Design review of the part built by this model. Coordinates are the model's own, in mm. A direction names the side the tool comes from. Give positions to 0.01 mm unless a question says otherwise; leave off trailing zeros. Write each loop counter-clockwise with the first axis right and the second up, starting at its lowest first coordinate (ties: lowest second). Pieces come first, ordered by that corner, then holes. Notation, with made-up numbers: M -27,56 L -12,56 A19 ccw -12,90 Z; hole C 42.5,7 d11. An arc over 180 degrees is marked long. Use a Markdown table: item, result. Add a question column.
Autodesk Inventor part; units mm, degrees
ref_plane "Start plane" through (0, 0, 0) normal (0, 0, 1) x (1, 0, 0)
ref_plane "End plane" through (0, 0, 685) normal (0, 0, 1) x (1, 0, 0)
ref_plane "Work Plane4" through (0, 0, 342.5) normal (-1, 0, 0) x (0, 0, 1)
ref_plane "Start plane" through (0, 0, 0) normal (0, 0, 1) x (1, 0, 0)
ref_plane "End plane" through (0, 0, 685) normal (0, 0, 1) x (1, 0, 0)
sketch "Sketch" plane through (0, 0, 0) normal (0, 0, 1) x (1, 0, 0)
  line L0 (-17.5, -13.5) -> (-17.5, 13.5)
  line L1 (-13.5, 17.5) -> (13.5, 17.5)
  line L2 (17.5, 13.5) -> (17.5, -13.5)
  line L3 (13.5, -17.5) -> (-13.5, -17.5)
  arc A0 (-17.5, -13.5) -> (-13.5, -17.5) centre (-13.5, -13.5) ccw
  arc A1 (-13.5, 17.5) -> (-17.5, 13.5) centre (-13.5, 13.5) ccw
  arc A2 (17.5, 13.5) -> (13.5, 17.5) centre (13.5, 13.5) ccw
  arc A3 (13.5, -17.5) -> (17.5, -13.5) centre (13.5, -13.5) ccw
  arc A4 (-13.5, 15.5) -> (-15.5, 13.5) centre (-13.5, 13.5) ccw
  line L4 (-13.5, 15.5) -> (13.5, 15.5)
  arc A5 (15.5, 13.5) -> (13.5, 15.5) centre (13.5, 13.5) ccw
  line L5 (15.5, 13.5) -> (15.5, -13.5)
  arc A6 (13.5, -15.5) -> (15.5, -13.5) centre (13.5, -13.5) ccw
  line L6 (13.5, -15.5) -> (-13.5, -15.5)
  arc A7 (-15.5, -13.5) -> (-13.5, -15.5) centre (-13.5, -13.5) ccw
  line L7 (-15.5, -13.5) -> (-15.5, 13.5)
  line L8 (0, 25.6598) -> (0, -25.6598) construction
  line L9 (-25.6598, 0) -> (25.6598, 0) construction
  dimension "d7" = 4
  dimension "d10" = 35
  dimension "d11" = 35
  dimension "d12" = 2
  dimension "d15" = 17.5
  dimension "d16" = 17.5
extrude "Body" add sketch "Sketch" along normal up to surface (685 mm away) from surface at 0
sketch "Sketch3" plane through (0, 0, 0) normal (0, 0, 1) x (1, 0, 0)
  line L0 (0, 0) -> (10, 0)
ref_plane "Work Plane3" through (0, 0, 0) normal (0, -1, 0) x (1, 0, 0)
sketch "Sketch4" plane through (0, 0, 0) normal (0, -1, 0) x (1, 0, 0)
  line L0 (-2, 0) -> (12, 0)
  line L1 (-2, 685) -> (12, 685)
  dimension "d18" = 685
ref_plane "Work Plane4" through (0, 0, 342.5) normal (-1, 0, 0) x (0, 0, 1)
ref_plane "Work Plane5" through (-395, 0, 342.5) normal (-1, 0, 0) x (0, 0, 1)
ref_plane "Work Plane6" through (-197.5, 0, 342.5) normal (-1, 0, 0) x (0, 0, 1)
sketch "Sketch5" plane through (-197.5, 0, 342.5) normal (-1, 0, 0) x (0, 0, 1)
  arc A0 (-17.5, -13.5) -> (-13.5, -17.5) centre (-13.5, -13.5) ccw
  line L0 (-17.5, -13.5) -> (-17.5, 13.5)
  arc A1 (-13.5, 17.5) -> (-17.5, 13.5) centre (-13.5, 13.5) ccw
  line L1 (-13.5, 17.5) -> (13.5, 17.5)
  arc A2 (17.5, 13.5) -> (13.5, 17.5) centre (13.5, 13.5) ccw
  line L2 (17.5, 13.5) -> (17.5, -13.5)
  arc A3 (13.5, -17.5) -> (17.5, -13.5) centre (13.5, -13.5) ccw
  line L3 (13.5, -17.5) -> (-13.5, -17.5)
  arc A4 (-13.5, 15.5) -> (-15.5, 13.5) centre (-13.5, 13.5) ccw
  line L4 (-13.5, 15.5) -> (13.5, 15.5)
  arc A5 (15.5, 13.5) -> (13.5, 15.5) centre (13.5, 13.5) ccw
  line L5 (15.5, 13.5) -> (15.5, -13.5)
  arc A6 (13.5, -15.5) -> (15.5, -13.5) centre (13.5, -13.5) ccw
  line L6 (13.5, -15.5) -> (-13.5, -15.5)
  arc A7 (-15.5, -13.5) -> (-13.5, -15.5) centre (-13.5, -13.5) ccw
  line L7 (-15.5, -13.5) -> (-15.5, 13.5)
extrude "Extrusion2" cut sketch "Sketch5" along normal up to surface (395 mm away) from surface at -197.5 contours L0 A1 L1 A2 L2 A3 L3 A0 | L4 A5 L5 A6 L6 A7 L7 A4
equation "\"d7\" = G_IR"
equation "\"d10\" = G_H"
equation "\"d11\" = G_W"
equation "\"d12\" = G_T"
equation "\"d15\" = 0.5 * d10"
equation "\"d16\" = 0.5 * d11"
equation "\"d3\" = G_L"
equation "\"G_W\" = 35"
equation "\"G_H\" = 35"
equation "\"G_T\" = 2"
equation "\"G_IR\" = 4"
equation "\"G_L\" = d18"
equation "\"G_OFFSET_START\" = 0"
equation "\"G_OFFSET_END\" = 0"
equation "\"d14\" = G_OFFSET_END + B_L"
equation "\"B_L\" = 685"
properties part number "AS 1163 - C350L0 35x35x2.0 SHS - 685" material "Steel, Mild"
(1) Add section C-C on z = 191. Give the boundary of the cut face in (x, y), then the cut area to 3 significant figures.
(2) For pin 1 (1.6 mm diameter, centred on y = -17, z = 336.5, fed in from -X); pin 2 (1 mm diameter, centred on x = -16, y = 5, fed in from -Z); pin 3 (5 mm diameter, centred on y = 5, z = 350, fed in from -X), all flat-tipped, find the tip position at first contact; note any pin that passes through.
(3) Add section B-B on x = 8. Give the boundary of the cut face in (y, z), then the cut area to 3 significant figures.
(4) Add section A-A on y = -0.5. Give the boundary of the cut face in (x, z).
(5) The part is to be moulded in two halves that separate along Y. For faces 3 (the flat face through (-16, 3, 0)), 4 (the flat face through (3, 17.5, 338)), 5 (the flat face through (0.2, -15.5, 337.7)), say which applies: released by +Y, released by -Y, zero draft, split by the parting line, or undercut.
(6) Machinability: for faces 1 (the flat face through (-17.5, 0, 520)), 2 (the flat face through (15.5, 0, 338)), which of the approach directions +Z, -Z, +X, -X, +Y, -Y give a long, thin tool a straight path to every point of the face, cutting with its end or side? Answer none if there is none.
(7) Wall thickness on L1, parallel to X at y = 7.5, z = 149.5; L2, parallel to X at y = 14, z = 202: over which ranges is each line inside the solid? List them lowest first.
From the geometry:
| question | item | result |
|---|---|---|
| 1 | outline | M -17.5,-13.5 A4 ccw -13.5,-17.5 L 13.5,-17.5 A4 ccw 17.5,-13.5 L 17.5,13.5 A4 ccw 13.5,17.5 L -13.5,17.5 A4 ccw -17.5,13.5 Z; hole M -15.5,-13.5 A2 ccw -13.5,-15.5 L 13.5,-15.5 A2 ccw 15.5,-13.5 L 15.5,13.5 A2 ccw 13.5,15.5 L -13.5,15.5 A2 ccw -15.5,13.5 Z |
| 1 | area | 254 mm^2 |
| 2 | pin 1 | stops at x = 0 |
| 2 | pin 2 | stops at z = 0 |
| 2 | pin 3 | stops at x = 15.5 |
| 3 | outline | M -17.5,0 L -15.5,0 L -15.5,685 L -17.5,685 Z; M 15.5,0 L 17.5,0 L 17.5,685 L 15.5,685 Z |
| 3 | area | 2,740 mm^2 |
| 4 | outline | M -17.5,0 L -15.5,0 L -15.5,325 L -17.5,325 Z; M -17.5,360 L -15.5,360 L -15.5,685 L -17.5,685 Z; M 15.5,0 L 17.5,0 L 17.5,685 L 15.5,685 Z |
| 5 | face 3 | zero draft |
| 5 | face 4 | released by +Y |
| 5 | face 5 | undercut |
| 6 | face 1 | +Z, -Z, -X, +Y, -Y |
| 6 | face 2 | +Z, -Z |
| 7 | L1 | x = -17.5 to -15.5, 15.5 to 17.5 |
| 7 | L2 | x = -17.47 to -15.44, 15.44 to 17.47 |
